from build123d import *

# Parameters (mm, degrees)
SKETCH_1_W      = 20
SKETCH_1_H      = 16
EXTRUDE_1_DEPTH = 8
SKETCH_2_R      = 6
EXTRUDE_2_DEPTH = 2
SKETCH_3_R      = 4
EXTRUDE_3_DEPTH = 4
SKETCH_4_R      = 3
EXTRUDE_4_DEPTH = 4


with BuildPart() as part:
    # 草图1 → 凸台-拉伸1 (new body, symmetric)
    with BuildSketch(Plane(origin=(0, 0, 0), x_dir=(1, 0, 0), z_dir=(0, 1, 0))):
        Rectangle(SKETCH_1_W, SKETCH_1_H)
    extrude(amount=EXTRUDE_1_DEPTH, both=True)

    # 草图2 → 凸台-拉伸2 (add)
    with BuildSketch(Plane(origin=(0, 0, -8), x_dir=(-1, 0, 0), z_dir=(0, 0, -1))):
        Circle(SKETCH_2_R)
    extrude(amount=EXTRUDE_2_DEPTH)

    # 草图3 → 凸台-拉伸3 (add)
    with BuildSketch(Plane.XZ.offset(8)):
        Circle(SKETCH_3_R)
    extrude(amount=EXTRUDE_3_DEPTH)

    # 草图4 → 凸台-拉伸4 (add)
    with BuildSketch(Plane(origin=(0, 8, 0), x_dir=(1, 0, 0), z_dir=(0, 1, 0))):
        Circle(SKETCH_4_R)
    extrude(amount=EXTRUDE_4_DEPTH)


solid = part.part
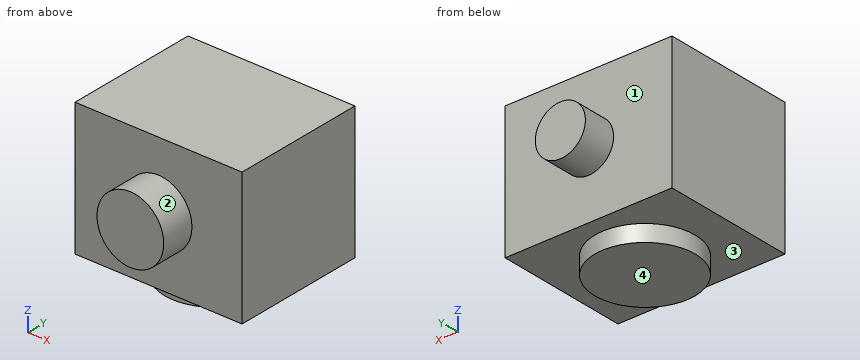
Can you work these out from the model? Positions are in its coordinate system, mm. Face numbers are marked on the shaded views. A direction names the side the tool comes from. Round coordinates to 2 decimals unless told otherwise and drop trailing zeros. Order: outer loops, then holes, each group sorted by start corner. A loop starts at its lowest first (then second) coordinate and runs counter-clockwise, first axis right, second up. Notation, with made-up numbers: M 58.5,-24 L 98.5,-24 A21 cw 98.5,-14 Z; hole C 86,73 d6. An arc over 180 degrees is marked long. Use a Markdown table: item, result.
1) I'm going to push a flat-ended pin straight in: P1, Ø3, axis at x = 6.5, z = 0, coming from the -Y side. Where does the tip first touch, or does it pass through?
Geometry says:
| item | result |
|---|---|
| P1 | stops at y = -8 |
2) Imagine slicing it at D-D (x = -5). List the corners of the cut face in (y, z) for me, then the cut area to 3 significant figures.
Geometry says:
| item | result |
|---|---|
| outline | M -8,-8 L -3.32,-8 L -3.32,-10 L 3.32,-10 L 3.32,-8 L 8,-8 L 8,8 L -8,8 Z |
| area | 269 mm² |
3) Imagine slicing it at B-B (x = 0). List the corners of the cut face in (y, z) for me.
Geometry says:
| item | result |
|---|---|
| outline | M -12,-4 L -8,-4 L -8,-8 L -6,-8 L -6,-10 L 6,-10 L 6,-8 L 8,-8 L 8,-3 L 12,-3 L 12,3 L 8,3 L 8,8 L -8,8 L -8,4 L -12,4 Z |
4) On a 3-axis mill with a long thin cutter (end or side, diameter ignored), from which of +Z, -Z, +X, -X, +Y, -Y can I reach the whole of each face in a straight line? I mean the marked faces 1, 2, 3 and 4. Say none if no direction works.
Geometry says:
| item | result |
|---|---|
| face 1 | +Y |
| face 2 | -Y |
| face 3 | -Z |
| face 4 | -Z, +X, -X, +Y, -Y |
5) If I drill on line 1 along Y through (x, z) = (0.5, -3); line 2 along Z through (x, y) = (6.75, 0.5), over which ranges is the centre line in solid material (lowest first)?
Geometry says:
| item | result |
|---|---|
| line 1 | y = -12 to 8 |
| line 2 | z = -8 to 8 |
